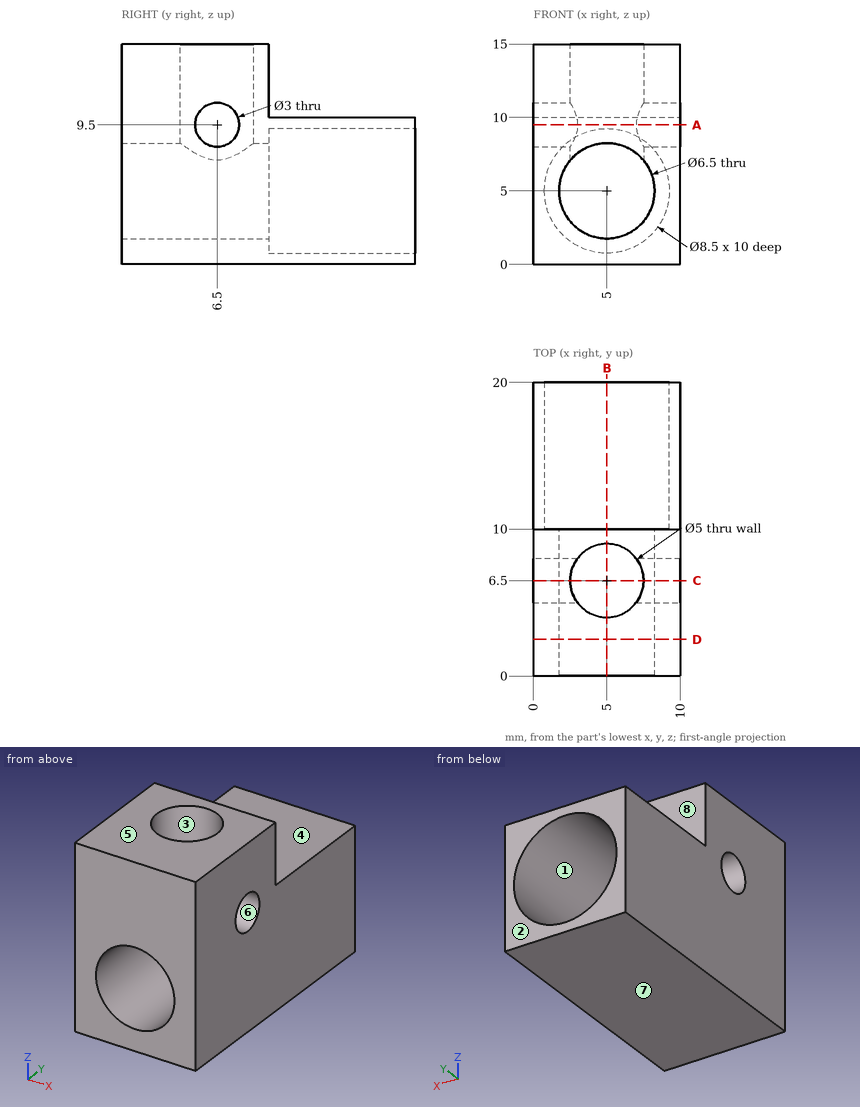
Verification items for this drawing (mm, ordinates from the low corner). A direction names the side the tool comes from. Give positions to 0.01 mm unless a question says otherwise; leave off trailing zeros. Loops run counter-clockwise (first coordinate to the right, second up) from the corner with the lowest first, then second, coordinate; pieces in that order, holes last. Notation, with made-up numbers: M 17.5,51 L 63.5,51 A27 ccw 63.5,89 Z; hole C -2,41.25 d7. An arc over 180 degrees is marked long. Write item = value, one per line.
(1) Sectioned sample at D-D, the plane y = 2.5. Record the cut outline in (x, z), plus the area to 3 significant figures.
Answer below:
outline = M 0,0 L 10,0 L 10,15 L 0,15 Z; hole C 5,5 d6.5
area = 117 mm2
(2) Gauge pin test, flat ends, axial feed: pin 1 Ø5 at (x, y) = (5, 14) entering from +Z; pin 2 Ø1.5 at (x, z) = (5.5, 13.5) entering from +Y. Record the tip position at first contact, or that the pin passes through.
Answer below:
pin_1 = 10
pin_2 = 10
(3) Sectioned sample at B-B, the plane x = 5. Record the cut outline in (y, z).
Answer below:
outline = M 0,0 L 20,0 L 20,0.75 L 10,0.75 L 10,1.75 L 0,1.75 Z; M 0,8.25 L 4,8.25 L 4,15 L 0,15 Z; M 9,8.25 L 10,8.25 L 10,9.25 L 20,9.25 L 20,10 L 10,10 L 10,15 L 9,15 Z
(4) Tool access check on the marked faces 1, 2, 3, 4 and 5. Record the directions out of +Z, -Z, +X, -X, +Y, -Y that give a thin tool (end or side, any length) a straight path to the whole face; none if there is none.
Answer below:
face_1 = +Y
face_2 = +Z, -Z, +X, -X, +Y
face_3 = +Z
face_4 = +Z, +X, -X, +Y
face_5 = +Z, +X, -X, +Y, -Y
(5) Material ranges on line 1 (Y direction, x = 5, z = 13.25); line 2 (Y direction, x = 5, z = 9.5); line 3 (Z direction, x = 5, y = 13.75), recorded low to high. Write a range as [from, to].
Answer below:
line_1 = [0, 4], [9, 10]
line_2 = [0, 4], [9, 20]
line_3 = [0, 0.75], [9.25, 10]
(6) Sectioned sample at C-C, the plane y = 6.5. Record the cut outline in (x, z).
Answer below:
outline = M 0,0 L 10,0 L 10,8 L 7.5,8 L 7.5,7.08 A3.25 cw long 2.5,7.08 L 2.5,8 L 0,8 Z; M 0,11 L 2.5,11 L 2.5,15 L 0,15 Z; M 7.5,11 L 10,11 L 10,15 L 7.5,15 Z
(7) Sectioned sample at A-A, the plane z = 9.5. Record the cut outline in (x, y), plus the area to 3 significant figures.
Answer below:
outline = M 0,0 L 10,0 L 10,5 L 7,5 A2.5 cw 3,5 L 0,5 Z; M 0,8 L 3,8 A2.5 cw 7,8 L 10,8 L 10,20 L 0,20 Z
area = 164 mm2
(8) Release check for a two-part mould opening along Z. For the marked faces 6, 7 and 8 record: released by +Z, released by -Z, zero draft, split by the parting line, or undercut.
Answer below:
face_6 = undercut
face_7 = released by -Z
face_8 = zero draft
